Could you check a few things on this model? Use its own coordinates, in mm. Face numbers are marked on the shaded views. A direction names the side the tool comes from. Round coordinates to 2 decimals unless told otherwise and drop trailing zeros. Write each loop counter-clockwise with the first axis right and the second up, starting at its lowest first coordinate (ties: lowest second). Pieces come first, ordered by that corner, then holes.
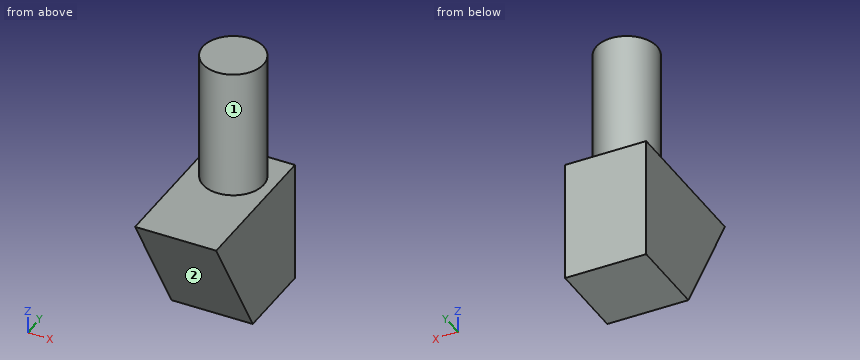
```python
from build123d import *

# Parameters (mm, degrees)
F0_W     = 6.35
F0_H     = 6.35
F1_DEPTH = 9.525
F2_R     = 2.3749
F3_DEPTH = 10.16
F5_DEPTH = 6.35


with BuildPart() as f1:
    # F0 (on Top) → F1 (new body)
    with BuildSketch(Plane.XY):
        with Locations((3.175, 3.175)):
            Rectangle(F0_W, F0_H)
    extrude(amount=F1_DEPTH)

    # F2 (on face) → F3 (join)
    with BuildSketch(Plane.XY.offset(9.525)):
        with Locations((3.175, 3.175)):
            Circle(F2_R)
    extrude(amount=F3_DEPTH)

    # F4 (on face) → F5 (join, through all)
    with BuildSketch(Plane(origin=(0, 0, 0), x_dir=(0, -1, 0), z_dir=(-1, 0, 0))):
        Polygon((5.499261, 9.525), (0, 9.525), (0, 0), align=None)
    extrude(amount=-F5_DEPTH)


solid = f1.part
```
Q1. If I drill on L1, parallel to Z at x = 2.5, y = 5.75 (3 decimals); L2, parallel to X at y = 3.25, z = 16.5, over which ranges is the centre line in solid material (lowest first)?
Q2. Imagine slicing it at A-A, the plane x = 3.5. Write out the boundary of the cut face in (y, z) (3 decimals).
Q3. Imagine slicing it at B-B, the plane y = 0.5. Write out the boundary of the cut face in (x, z) (3 decimals), then the cut area to 3 significant figures.
Q4. On a 3-axis mill with a long thin cutter (end or side, diameter ignored), from which of +Z, -Z, +X, -X, +Y, -Y can I reach the whole of each face in a straight line? I mean the marked faces 1 and 2. Say none if no direction works.
Q5. Imagine slicing it at C-C, the plane z = 16.25. Write out the boundary of the cut face in (x, y) (3 decimals), then the cut area to 3 significant figures.
Q6. I'm going to push flat-ended pins straight in: pin 1 Ø5 at (y, z) = (-2, 17) entering from +X; pin 2 Ø3 at (x, z) = (3, 17) entering from -Y. Where does each tip first touch, or does it pass through?
Q7. Imagine slicing it at D-D, the plane x = 5.75. Write out the boundary of the cut face in (y, z) (3 decimals).
Results found:
1. L1: z = 0 to 9.525
1. L2: x = 0.8 to 5.55
2. outline: (-5.499, 9.525) - (0, 0) - (6.35, 0) - (6.35, 9.525) - (5.528, 9.525) - (5.528, 19.685) - (0.822, 19.685) - (0.822, 9.525) - close
3. outline: (0, 0) - (6.35, 0) - (6.35, 9.525) - (0, 9.525) - close
3. area: 60.5 mm2
4. face 1: +Z
4. face 2: -Z, +X, -X, -Y
5. outline: circle Ø4.75 at (3.175, 3.175)
5. area: 17.7 mm2
6. pin 1: passes through
6. pin 2: stops at y = 0.8
7. outline: (-5.499, 9.525) - (0, 0) - (6.35, 0) - (6.35, 9.525) - close
